Part model, mm, in its own coordinate system. A direction names the side the tool comes from. Round coordinates to 2 decimals unless told otherwise and drop trailing zeros. Write each loop counter-clockwise with the first axis right and the second up, starting at its lowest first coordinate (ties: lowest second). Pieces come first, ordered by that corner, then holes. Notation, with made-up numbers: M 10,-33 L 48,-33 A24 cw 48,5 Z; hole C 64.5,73 d5. An arc over 180 degrees is marked long. Answer as a JSON object with one key per item and string values. Group by question number.
1. Drop flat-ended pins along their axis: pin 1 (1.5 mm diameter, centred on y = -6, z = 7.5, fed in from -X); pin 2 (9.5 mm diameter, centred on x = 0, y = 23.75, fed in from -Z); pin 3 (2 mm diameter, centred on y = 10, z = 13, fed in from +X); pin 4 (1.5 mm diameter, centred on x = -13, z = 3, fed in from -Y) (3 decimals). Give the stop position or say it passes through.
2. Band-saw the part on A-A, the plane x = 0. Write the cut outline in (y, z) (1 decimal).
3. Which spindle directions (+Z, -Z, +X, -X, +Y, -Y) get a long thin tool onto all of the face, cutting with end or side? Do faces 1 (the face through (18.19, -13.7, 8.11)), 2 (the face through (-3.79, -17.09, 9.1)). Say none if no direction does.
4. Band-saw the part on D-D, the plane y = 22.5. Write the cut outline in (x, z).
5. Drill centre lines: line 1 (Y direction, x = 0, z = 6) (1 decimal); line 2 (Y direction, x = 0, z = 0.95); line 3 (X direction, y = -11.5, z = 14.5). Where is each one in solid material? Low to high. Write a range as from..to.
6. Band-saw the part on B-B, the plane y = 0. Write the cut outline in (x, z) (3 decimals).
7. Band-saw the part on C-C, the plane x = -10.5. Write the cut outline in (y, z), plus the area to 3 significant figures.
8. Two-plate mould, pull along Y, no slides. Class faces 3 (the face through (-7, -14, 2)), 4 (the face through (-29.97, 1.32, 7.89)), 5 (the face through (13, -13, 16)): +Y half, -Y half, draft (parallel to the pull), parting line (faces both ways), or undercut.
from build123d import *

# Parameters (mm, degrees)
SKETCH1_R           = 30
BOSS_EXTRUDE1_DEPTH = 16
SKETCH2_R           = 17.505
CUT_EXTRUDE1_DEPTH  = 14
SKETCH4_R           = 15.5
CUT_EXTRUDE2_DEPTH  = 45.676615807
SKETCH5_R           = 3
CUT_EXTRUDE3_DEPTH  = 46.343136195


with BuildPart() as part:
    # Sketch1 → Boss-Extrude1 (new body)
    with BuildSketch(Plane.XY):
        Circle(SKETCH1_R)
    extrude(amount=BOSS_EXTRUDE1_DEPTH)

    # Sketch2 → Cut-Extrude1 (cut)
    with BuildSketch(Plane.XY.offset(16)):
        Circle(SKETCH2_R)
    extrude(amount=-CUT_EXTRUDE1_DEPTH, mode=Mode.SUBTRACT)

    # Sketch4 → Cut-Extrude2 (cut, through all)
    with BuildSketch(Plane.XY.offset(2)):
        Circle(SKETCH4_R)
    extrude(amount=-CUT_EXTRUDE2_DEPTH, mode=Mode.SUBTRACT)

    # Sketch5 → Cut-Extrude3 (cut, through all)
    with BuildSketch(Plane.XY.offset(16)):
        with Locations((0, 23.7525)):
            Circle(SKETCH5_R)
        with Locations((20.570268403, -11.87625)):
            Circle(SKETCH5_R)
        with Locations((-20.570268403, -11.87625)):
            Circle(SKETCH5_R)
    extrude(amount=-CUT_EXTRUDE3_DEPTH, mode=Mode.SUBTRACT)


solid = part.part
Worked answers:
{
 "1": {"pin 1": "stops at x = -29.54", "pin 2": "stops at z = 0", "pin 3": "stops at x = 28.62", "pin 4": "stops at y = -27.385"},
 "2": {"outline": "M -30,0 L -15.5,0 L -15.5,2 L -17.5,2 L -17.5,16 L -30,16 Z; M 15.5,0 L 20.8,0 L 20.8,16 L 17.5,16 L 17.5,2 L 15.5,2 Z; M 26.8,0 L 30,0 L 30,16 L 26.8,16 Z"},
 "3": {"face 1": "+Z, -Z", "face 2": "+Z"},
 "4": {"outline": "M -19.84,0 L -2.73,0 L -2.73,16 L -19.84,16 Z; M 2.73,0 L 19.84,0 L 19.84,16 L 2.73,16 Z"},
 "5": {"line 1": "y = -30..-17.5, 17.5..20.8, 26.8..30", "line 2": "y = -30..-15.5, 15.5..20.75, 26.75..30", "line 3": "x = -27.71..-23.55, -17.59..-13.2, 13.2..17.59, 23.55..27.71"},
 "6": {"outline": "M -30,0 L -15.5,0 L -15.5,2 L -17.505,2 L -17.505,16 L -30,16 Z; M 15.5,0 L 30,0 L 30,16 L 17.505,16 L 17.505,2 L 15.5,2 Z"},
 "7": {"outline": "M -28.1,0 L -11.4,0 L -11.4,2 L -14.01,2 L -14.01,16 L -28.1,16 Z; M 11.4,0 L 28.1,0 L 28.1,16 L 14.01,16 L 14.01,2 L 11.4,2 Z", "area": "461 mm^2"},
 "8": {"face 3": "undercut", "face 4": "parting line", "face 5": "draft"}
}
